Geometry check sheet. Reference: drawing and pictorial views, mm from the part's lowest x, y, z. Round coordinates to 2 decimals unless told otherwise and drop trailing zeros. Write each loop counter-clockwise with the first axis right and the second up, starting at its lowest first coordinate (ties: lowest second). Pieces come first, ordered by that corner, then holes. Notation, with made-up numbers: (11, 34.5) - (30, 34.5) arc R19 cw to (30, 45.5) - close; hole circle Ø1 at (79.25, -23). An arc over 180 degrees is marked (long way). Use one line per item in the form item = value. Start each with the question number.
1) Scan lines: probe 1 along Y at (x, z) = (65, 3); probe 2 along X at (y, z) = (23.5, 6); probe 3 along Z at (x, y) = (52.5, 14.75). Record each from-to range of solid material in increasing order.
2) Gauge pin test, flat ends, axial feed: P1, Ø1.2, axis at x = 64, y = 8, coming from the -Z side; P2, Ø6, axis at y = 7.5, z = 5, coming from the +X side; P3, Ø8, axis at y = 21, z = 4.5, coming from the -X side. Record the tip position at first contact, or that the pin passes through.
3) Section check D-D (y = 17.5). Record the boundary of the cut face in (x, z).
4) Draft check along X on the marked faces 1 and 2. Enter one of: +X half, -X half, draft (parallel to the pull), parting line (faces both ways), or undercut.
5) Section check C-C (x = 37). Record the boundary of the cut face in (y, z), then the cut area to 3 significant figures.
6) Section check A-A (z = 9.75). Record the boundary of the cut face in (x, y), then the cut area to 3 significant figures.
7) Section check B-B (y = 7.5). Record the boundary of the cut face in (x, z), then the cut area to 3 significant figures.
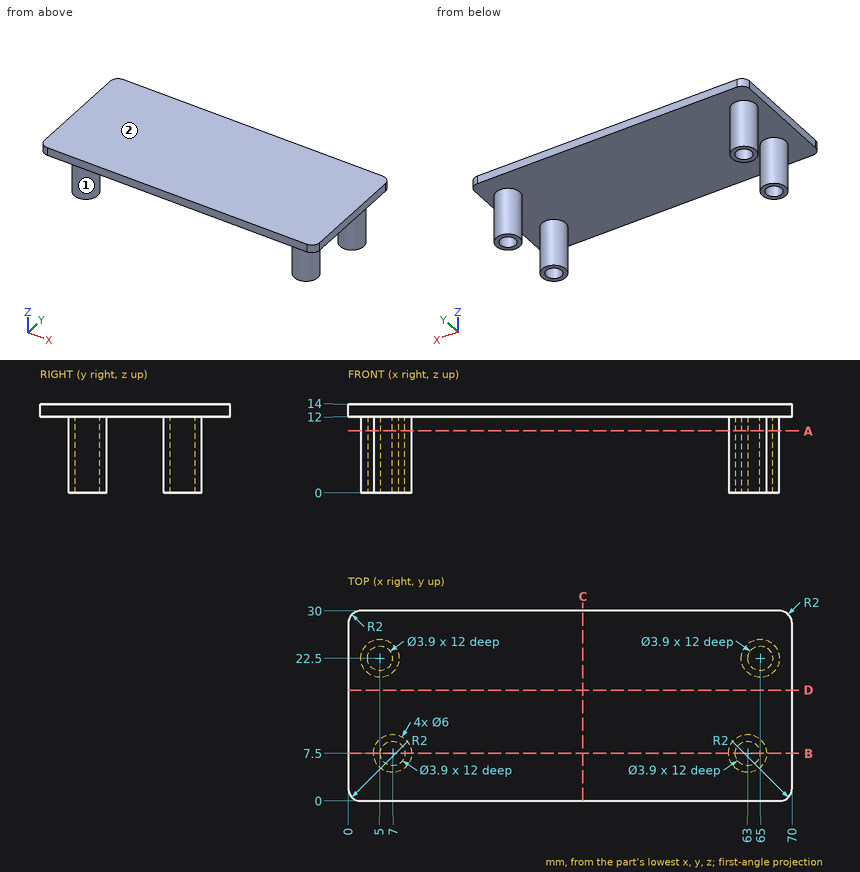
Results are:
q1.probe_1 = 5.26 to 9.74, 19.5 to 20.55, 24.45 to 25.5
q1.probe_2 = 2.17 to 3.33, 6.67 to 7.83, 62.17 to 63.33, 66.67 to 67.83
q1.probe_3 = 12 to 14
q2.P1 = 12
q2.P2 = 66
q2.P3 = 2
q3.outline = (0, 12) - (70, 12) - (70, 14) - (0, 14) - close
q4.face_1 = undercut
q4.face_2 = draft
q5.outline = (0, 12) - (30, 12) - (30, 14) - (0, 14) - close
q5.area = 60.0 mm²
q6.outline = circle Ø6 at (5, 22.5); circle Ø6 at (7, 7.5); circle Ø6 at (63, 7.5); circle Ø6 at (65, 22.5); hole circle Ø3.9 at (5, 22.5); hole circle Ø3.9 at (7, 7.5); hole circle Ø3.9 at (63, 7.5); hole circle Ø3.9 at (65, 22.5)
q6.area = 65.3 mm²
q7.outline = (0, 12) - (4, 12) - (4, 0) - (5.05, 0) - (5.05, 12) - (8.95, 12) - (8.95, 0) - (10, 0) - (10, 12) - (60, 12) - (60, 0) - (61.05, 0) - (61.05, 12) - (64.95, 12) - (64.95, 0) - (66, 0) - (66, 12) - (70, 12) - (70, 14) - (0, 14) - close
q7.area = 190 mm²
